Drawing for the job (mm, zero at the part's lowest x, y, z). Coordinates: 2 decimals unless noted, no trailing zeros. Loops run counter-clockwise (first coordinate to the right, second up) from the corner with the lowest first, then second, coordinate; pieces in that order, holes last. Notation, with made-up numbers: (71, 31) - (127, 31) arc R16 cw to (127, 58) - close; hole circle Ø1 at (11, 32.25). An arc over 180 degrees is marked (long way). Put each result on its own line as item: value.
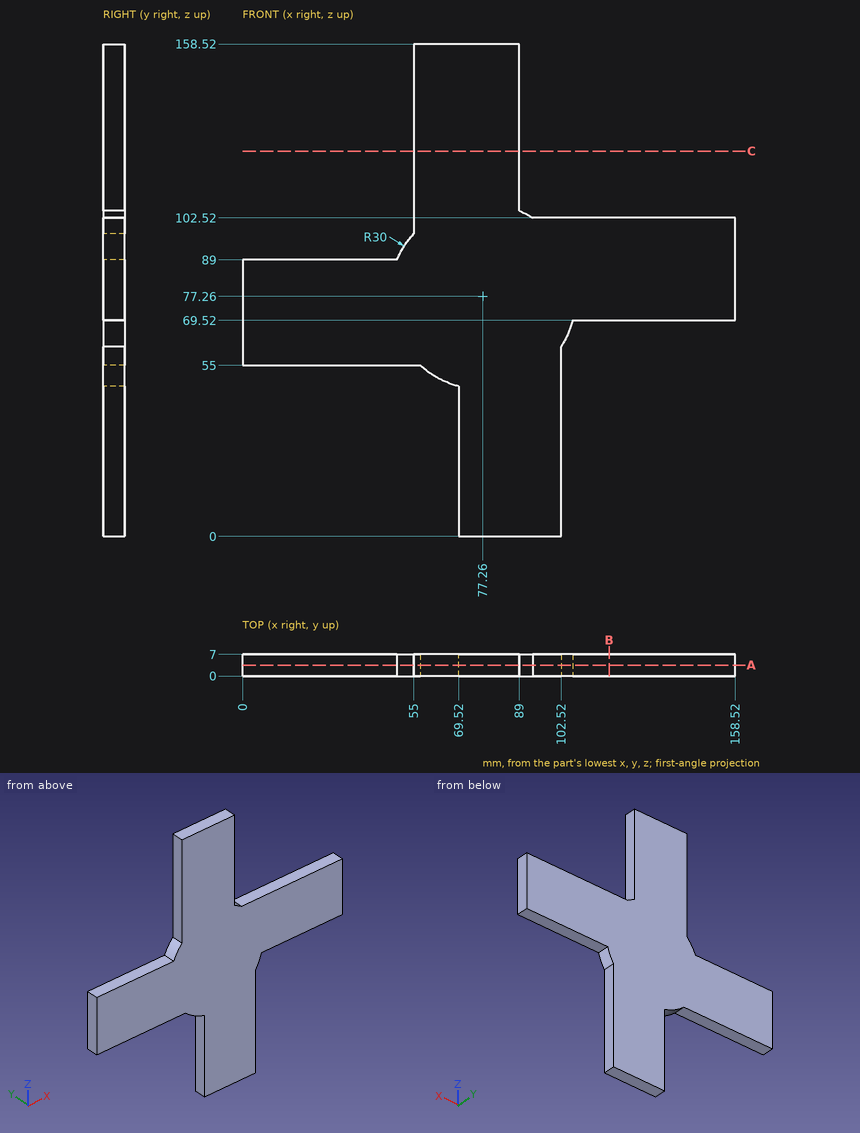
Q1. Pin check, flat tips, straight feed: pin 1 Ø3.5 at (y, z) = (2.5, 136.5) entering from -X; pin 2 Ø3.5 at (y, z) = (2, 34) entering from -X; pin 3 Ø2 at (x, y) = (32, 4.5) entering from +Z. Stop position of each tip, or through.
Determined:
pin 1: x = 55
pin 2: x = 69.52
pin 3: z = 89
Q2. Wall check: L1, parallel to Z at x = 28.5, y = 5.5; L2, parallel to X at y = 2.5, z = 59; L3, parallel to Z at x = 132.5, y = 4.75. Give the ranges that are in metal, low to high. Write a range as from..to.
Determined:
L1: 55..89
L2: 0..102.52
L3: 69.52..102.52
Q3. Slice it at C-C, the plane z = 124. Give the cut face in (x, y).
Determined:
outline: (55, 0) - (89, 0) - (89, 7) - (55, 7) - close
Q4. Slice it at A-A, the plane y = 3.5. Give the cut face in (x, z).
Determined:
outline: (0, 55) - (57.15, 55) arc R30 ccw to (69.52, 48.28) - (69.52, 0) - (102.52, 0) - (102.52, 61.08) arc R30 ccw to (106.24, 69.52) - (158.52, 69.52) - (158.52, 102.52) - (93.44, 102.52) arc R30 ccw to (89, 104.87) - (89, 158.52) - (55, 158.52) - (55, 97.37) arc R30 ccw to (49.65, 89) - (0, 89) - close
Q5. Slice it at B-B, the plane x = 118. Give the cut face in (y, z), then the cut area to 3 significant figures.
Determined:
outline: (0, 69.52) - (7, 69.52) - (7, 102.52) - (0, 102.52) - close
area: 231 mm2
